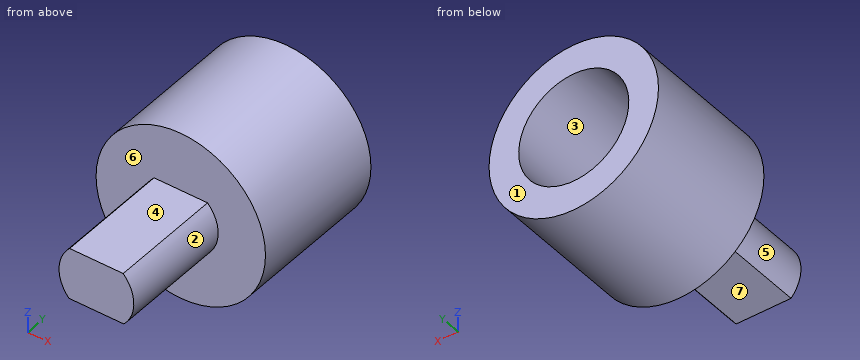
from build123d import *

# Parameters (mm, degrees)
SKETCH1_R           = 6
BOSS_EXTRUDE1_DEPTH = 2
SKETCH2_R           = 6
SKETCH2_R_2         = 3.9
BOSS_EXTRUDE2_DEPTH = 8
BOSS_EXTRUDE3_DEPTH = 8


with BuildPart() as part:
    # Sketch1 → Boss-Extrude1 (new body)
    with BuildSketch(Plane(origin=(0, 0, 0), x_dir=(1, 0, 0), z_dir=(0, 1, 0))):
        with Locations(Location((0, 0, 0), (0, 0, 270))):
            Circle(SKETCH1_R)
    extrude(amount=BOSS_EXTRUDE1_DEPTH)

    # Sketch2 → Boss-Extrude2 (add)
    with BuildSketch(Plane(origin=(0, 2, 0), x_dir=(1, 0, 0), z_dir=(0, 1, 0))):
        with Locations(Location((0, 0, 0), (0, 0, 270))):
            Circle(SKETCH2_R)
        with Locations(Location((0, 0, 0), (0, 0, 270))):
            Circle(SKETCH2_R_2, mode=Mode.SUBTRACT)
    extrude(amount=BOSS_EXTRUDE2_DEPTH)

    # Sketch3 → Boss-Extrude3 (add)
    with BuildSketch(Plane.XZ):
        with BuildLine():
            Line((-1.897366596, 1.85), (1.897366596, 1.85))
            ThreePointArc((1.897366596, 1.85), (2.649775646, 0.034482248), (1.944865034, -1.8))
            Line((1.944865034, -1.8), (-1.944865034, -1.8))
            ThreePointArc((-1.944865034, -1.8), (-2.649775646, 0.034482248), (-1.897366596, 1.85))
        make_face()
    extrude(amount=BOSS_EXTRUDE3_DEPTH)


solid = part.part
Part model, mm, in its own coordinate system. Face numbers are marked on the shaded views. A direction names the side the tool comes from. Coordinates: 2 decimals unless noted, no trailing zeros. Write each loop counter-clockwise with the first axis right and the second up, starting at its lowest first coordinate (ties: lowest second). Pieces come first, ordered by that corner, then holes. Notation, with made-up numbers: (-5.5, -4) - (53.5, -4) arc R26 cw to (53.5, 18) - close; hole circle Ø1 at (12, 37). An arc over 180 degrees is marked (long way). Put each result on its own line as item: value.
1. Two-plate mould, pull along X, no slides. Class the marked faces 1, 2 and 3: +X half, -X half, draft (parallel to the pull), parting line (faces both ways), or undercut.
Final values:
face 1: draft
face 2: +X half
face 3: undercut
2. Band-saw the part on B-B (y = 4.5). Write the cut outline in (x, z), then the cut area to 3 significant figures.
Final values:
outline: circle Ø12 at (0, 0); hole circle Ø7.8 at (0, 0)
area: 65.3 mm²
3. Band-saw the part on A-A (x = 0). Write the cut outline in (y, z).
Final values:
outline: (-8, -1.8) - (0, -1.8) - (0, -6) - (10, -6) - (10, -3.9) - (2, -3.9) - (2, 3.9) - (10, 3.9) - (10, 6) - (0, 6) - (0, 1.85) - (-8, 1.85) - close
4. Band-saw the part on C-C (z = 2.5). Write the cut outline in (x, y).
Final values:
outline: (-5.45, 0) - (5.45, 0) - (5.45, 10) - (2.99, 10) - (2.99, 2) - (-2.99, 2) - (-2.99, 10) - (-5.45, 10) - close
5. 3-axis set-ups, long thin cutter, end or side, ignore diameter. For the marked faces 4, 5, 6 and 7: which of +Z, -Z, +X, -X, +Y, -Y reach the whole face in a straight line?
Final values:
face 4: +Z, +X, -X, -Y
face 5: -X, -Y
face 6: -Y
face 7: -Z, +X, -X, -Y
6. Band-saw the part on D-D (y = 1). Write the cut outline in (x, z), then the cut area to 3 significant figures.
Final values:
outline: circle Ø12 at (0, 0)
area: 113 mm²
7. Flat gauge pins, fed straight in: pin 1 Ø1.5 at (x, z) = (-1.5, -4.5) entering from -Y; pin 2 Ø3 at (x, z) = (0.5, 2) entering from +Y; pin 3 Ø1.1 at (x, y) = (1, -2.5) entering from +Z. Where does each tip first touch, or does it go through?
Final values:
pin 1: stops at y = 0
pin 2: stops at y = 2
pin 3: stops at z = 1.85
8. Probe line 1 along X through (y, z) = (4.75, 0); line 2 along Y through (x, z) = (3, 5); line 3 along Y through (x, z) = (1.75, 1.5). List the from-to ranges inside material, lowest first. Write a range as [from, to].
Final values:
line 1: x = [-6, -3.9], [3.9, 6]
line 2: y = [0, 10]
line 3: y = [-8, 2]
